Input: part model. Units: mm. Frame: model coordinates. Face numbers are marked on the shaded views. Coordinates: 2 decimals unless noted, no trailing zeros. Loops run counter-clockwise (first coordinate to the right, second up) from the corner with the lowest first, then second, coordinate; pieces in that order, holes last. Notation, with made-up numbers: (22, 30.5) -> (63, 30.5) arc R21 ccw to (63, 51.5) -> close; hole circle Ø6 at (-5.5, -5). An arc over 180 degrees is marked (long way). Answer as a JSON object with one key per item and string values.
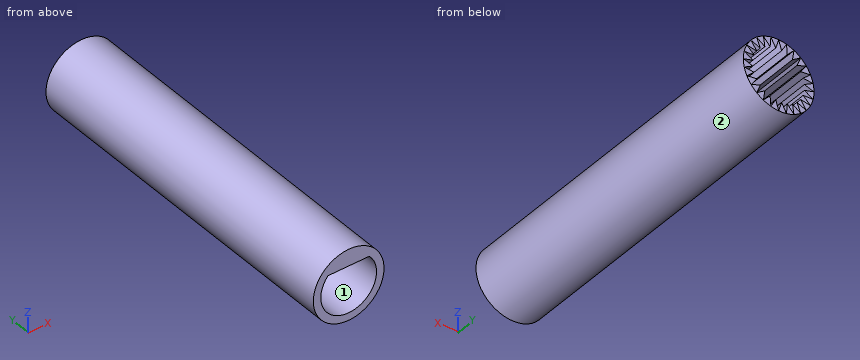
from build123d import *

# Parameters (mm, degrees)
SKETCH1_R           = 3.175
BOSS_EXTRUDE1_DEPTH = 18.000000068
SKETCH2_R           = 3.175
BOSS_EXTRUDE2_DEPTH = 0.254
SKETCH4_R           = 3.175
BOSS_EXTRUDE3_DEPTH = 12.7
CUT_EXTRUDE3_DEPTH  = 12.7


with BuildPart() as part:
    # Sketch1 → Boss-Extrude1 (new body)
    with BuildSketch(Plane(origin=(0, 0, 0), x_dir=(1, 0, 0), z_dir=(0, 1, 0))):
        with Locations(Location((0, 0, 0), (0, 0, 270))):
            Circle(SKETCH1_R)
        with BuildLine():
            Line((-1.855488288, -1.67829283), (1.855488288, -1.67829283))
            ThreePointArc((1.855488288, -1.67829283), (0, 2.5019), (-1.855488288, -1.67829283))
        make_face(mode=Mode.SUBTRACT)
    extrude(amount=BOSS_EXTRUDE1_DEPTH)

    # Sketch2 → Boss-Extrude2 (add)
    with BuildSketch(Plane(origin=(0, 18.000000068, 0), x_dir=(1, 0, 0), z_dir=(0, 1, 0))):
        with Locations(Location((0, 0, 0), (0, 0, 270))):
            Circle(SKETCH2_R)
    extrude(amount=BOSS_EXTRUDE2_DEPTH)

    # Sketch4 → Boss-Extrude3 (add)
    with BuildSketch(Plane(origin=(0, 18.254000068, 0), x_dir=(1, 0, 0), z_dir=(0, 1, 0))):
        with Locations(Location((0, 0, 0), (0, 0, 270))):
            Circle(SKETCH4_R)
    extrude(amount=BOSS_EXTRUDE3_DEPTH)

    # Sketch5 → Cut-Extrude3 (cut)
    with BuildSketch(Plane(origin=(0, 30.954000068, 0), x_dir=(1, 0, 0), z_dir=(0, 1, 0))):
        Polygon((0.703027733, 3.08016575), (0.260735719, 2.314093511), (0, 3.159377952), (-0.260735719, 2.314093511), (-0.703027733, 3.08016575), (-0.76913278, 2.1980552), (-1.370802719, 2.846501177), (-1.238962311, 1.971797222), (-1.969839933, 2.470101148), (-1.646665099, 1.646665099), (-2.470101148, 1.969839933), (-1.971797222, 1.238962311), (-2.846501177, 1.370802719), (-2.1980552, 0.76913278), (-3.08016575, 0.703027733), (-2.314093511, 0.260735719), (-3.159377952, 0), (-2.314093511, -0.260735719), (-3.08016575, -0.703027733), (-2.1980552, -0.76913278), (-2.846501177, -1.370802719), (-1.971797222, -1.238962311), (-2.470101148, -1.969839933), (-1.646665099, -1.646665099), (-1.969839933, -2.470101148), (-1.238962311, -1.971797222), (-1.370802719, -2.846501177), (-0.76913278, -2.1980552), (-0.703027733, -3.08016575), (-0.260735719, -2.314093511), (0, -3.159377952), (0.260735719, -2.314093511), (0.703027733, -3.08016575), (0.76913278, -2.1980552), (1.370802719, -2.846501177), (1.238962311, -1.971797222), (1.969839933, -2.470101148), (1.646665099, -1.646665099), (2.470101148, -1.969839933), (1.971797222, -1.238962311), (2.846501177, -1.370802719), (2.1980552, -0.76913278), (3.08016575, -0.703027733), (2.314093511, -0.260735719), (3.159377952, 0), (2.314093511, 0.260735719), (3.08016575, 0.703027733), (2.1980552, 0.76913278), (2.846501177, 1.370802719), (1.971797222, 1.238962311), (2.470101148, 1.969839933), (1.646665099, 1.646665099), (1.969839933, 2.470101148), (1.238962311, 1.971797222), (1.370802719, 2.846501177), (0.76913278, 2.1980552), align=None)
    extrude(amount=-CUT_EXTRUDE3_DEPTH, mode=Mode.SUBTRACT)


solid = part.part
1. Section query A-A (y = 14.5). Return loops of the section in (x, z) (3 decimals), plus the area to 3 significant figures.
Reply:
{"outline": "circle Ø6.35 at (0, 0); hole (-1.855, 1.678) arc R2.502 ccw (long way) to (1.855, 1.678) -> close", "area": "14.1 mm2"}
2. Mould query, pull axis Z, two halves, no side actions, for the marked faces 1 and 2. Classes: pulls with the +Z half, pulls with the -Z half, needs draft (parallel to the pull), parting line crosses it, or undercut.
Reply:
{"face 1": "undercut", "face 2": "parting line crosses it"}
3. Line query: line 1 along X through (y, z) = (8.5, 0) (3 decimals); line 2 along Y through (x, z) = (2.25, 1.25); line 3 along X through (y, z) = (17.5, 1). Output: solid intervals per line, ascending.
Reply:
{"line 1": "x = -3.175 to -2.502, 2.502 to 3.175", "line 2": "y = 0 to 18.25", "line 3": "x = -3.01 to -2.29, 2.29 to 3.01"}
